Geometry check sheet. Reference: the model listing, model coordinates, mm. Round coordinates to 2 decimals unless told otherwise and drop trailing zeros. Order: outer loops, then holes, each group sorted by start corner. A loop starts at its lowest first (then second) coordinate and runs counter-clockwise, first axis right, second up. Notation, with made-up numbers: (-2, 79) - (53, 79) arc R22 cw to (53, 107) - close; hole circle Ø5 at (38, 32). An arc over 180 degrees is marked (long way). Return JSON: item names as keys, results as strings. Group by question number.
Q1. Material ranges on line 1 along Y through (x, z) = (9.5, 0.25); line 2 along X through (y, z) = (18.5, 0.3) (3 decimals); line 3 along X through (y, z) = (13.5, 0.4) (3 decimals), recorded low to high.
Q2. Sectioned sample at A-A, the plane x = 29.5. Record the cut outline in (y, z), then the cut area to 3 significant figures.
Q3. Gauge pin test, flat end, axial feed: pin 1 Ø7.5 at (x, y) = (31.75, 15.875) entering from -Z. Record the tip position at first contact, or that the pin passes through.
Q4. Sectioned sample at D-D, the plane x = 38. Record the cut outline in (y, z), then the cut area to 3 significant figures.
Q5. Sectioned sample at B-B, the plane z = 0.55. Give the number of separate pieces and of enclosed holes in the cut face, then the cut area to 3 significant figures.
Q6. Draft check along Y on faces 1 (the flat face through (16, 16, 0)), 2 (the cylindrical face through (0.42, 12.65, 0.39)), 3 (the cylindrical face through (-5.903, 3.819, 0.394)). Enter one of: pulls with the +Y half, pulls with the -Y half, needs draft (parallel to the pull), parting line crosses it, or undercut.
Q7. Sectioned sample at C-C, the plane y = 25.5. Record the cut outline in (x, z).
```python
from build123d import *

# Parameters (mm, degrees)
SKETCH1_R           = 3.2512
BOSS_EXTRUDE1_DEPTH = 0.800000051
SKETCH3_R           = 0.4064
CUT_EXTRUDE3_DEPTH  = 53.080016562


with BuildPart() as part:
    # Sketch1 → Boss-Extrude1 (new body)
    with BuildSketch(Plane.XY):
        with BuildLine():
            Line((28.575, 31.75), (3.175, 31.75))
            ThreePointArc((3.175, 31.75), (-5.805256121, 28.030256121), (-9.525, 19.05))
            Line((-9.525, 19.05), (-9.525, 12.7))
            ThreePointArc((-9.525, 12.7), (-5.805256121, 3.719743879), (3.175, 0))
            Line((3.175, 0), (28.575, 0))
            ThreePointArc((28.575, 0), (37.555256121, 3.719743879), (41.275, 12.7))
            Line((41.275, 12.7), (41.275, 19.05))
            ThreePointArc((41.275, 19.05), (37.555256121, 28.030256121), (28.575, 31.75))
        make_face()
        with Locations(Location((0, 15.875, 0), (0, 0, 180))):
            Circle(SKETCH1_R, mode=Mode.SUBTRACT)
        with Locations(Location((31.75, 15.875, 0), (0, 0, 180))):
            Circle(SKETCH1_R, mode=Mode.SUBTRACT)
    extrude(amount=BOSS_EXTRUDE1_DEPTH)

    # Sketch3 → Cut-Extrude3 (cut, through all)
    with BuildSketch(Plane(origin=(0, 0, 0.800000051), x_dir=(-1, 0, 0), z_dir=(0, 0, -1))):
        with Locations((-14.605, 30.353)):
            Circle(SKETCH3_R)
        with Locations((-12.065, 30.353)):
            Circle(SKETCH3_R)
        with Locations((-9.525, 30.353)):
            Circle(SKETCH3_R)
        with Locations((-6.985, 30.353)):
            Circle(SKETCH3_R)
        with Locations(Location((-24.765, 30.353, 0), (0, 0, 180))):
            Circle(SKETCH3_R)
        with Locations(Location((-22.225, 30.353, 0), (0, 0, 180))):
            Circle(SKETCH3_R)
        with Locations(Location((-19.685, 30.353, 0), (0, 0, 180))):
            Circle(SKETCH3_R)
        with Locations(Location((-17.145, 30.353, 0), (0, 0, 180))):
            Circle(SKETCH3_R)
        with Locations((-17.145, 1.397)):
            Circle(SKETCH3_R)
        with Locations((-19.685, 1.397)):
            Circle(SKETCH3_R)
        with Locations((-22.225, 1.397)):
            Circle(SKETCH3_R)
        with Locations((-24.765, 1.397)):
            Circle(SKETCH3_R)
        with Locations(Location((-6.985, 1.397, 0), (0, 0, 180))):
            Circle(SKETCH3_R)
        with Locations(Location((-9.525, 1.397, 0), (0, 0, 180))):
            Circle(SKETCH3_R)
        with Locations(Location((-12.065, 1.397, 0), (0, 0, 180))):
            Circle(SKETCH3_R)
        with Locations(Location((-14.605, 1.397, 0), (0, 0, 180))):
            Circle(SKETCH3_R)
    extrude(amount=CUT_EXTRUDE3_DEPTH, mode=Mode.SUBTRACT)


solid = part.part
```
Reply:
{
 "1": {"line 1": "0 to 0.99, 1.8 to 29.95, 30.76 to 31.75", "line 2": "-9.525 to -1.918, 1.918 to 29.832, 33.668 to 41.275", "line 3": "-9.525 to -2.22, 2.22 to 29.53, 33.97 to 41.275"},
 "2": {"outline": "(0.03, 0) - (13.53, 0) - (13.53, 0.8) - (0.03, 0.8) - close; (18.22, 0) - (31.72, 0) - (31.72, 0.8) - (18.22, 0.8) - close", "area": "21.6 mm^2"},
 "3": {"pin 1": "z = 0"},
 "4": {"outline": "(4.19, 0) - (27.56, 0) - (27.56, 0.8) - (4.19, 0.8) - close", "area": "18.7 mm^2"},
 "5": {"separate pieces": "1", "enclosed holes": "18", "area": "1,400 mm^2"},
 "6": {"face 1": "needs draft", "face 2": "undercut", "face 3": "pulls with the -Y half"},
 "7": {"outline": "(-7.77, 0) - (39.52, 0) - (39.52, 0.8) - (-7.77, 0.8) - close"}
}
